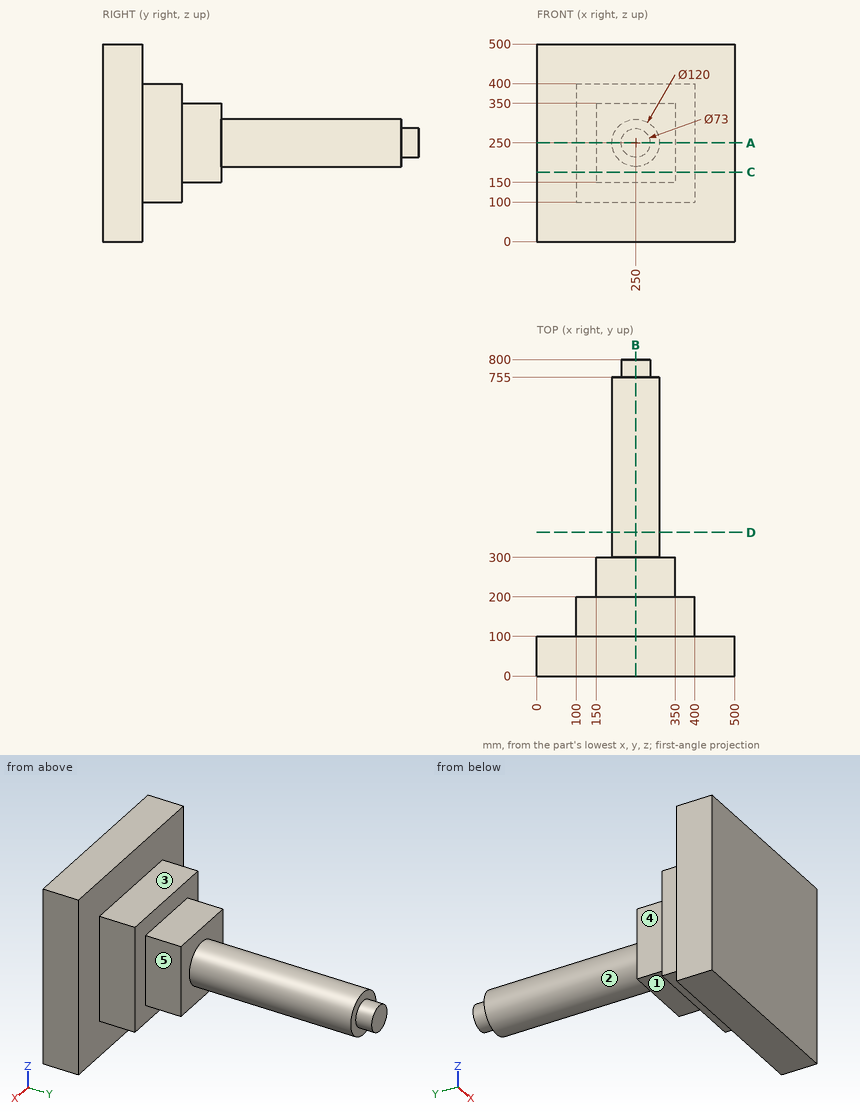
The drawing under review shows one solid part. Ordinate dimensions are in mm from its lowest x, y, z. A direction names the side the tool comes from. Give positions to 0.01 mm unless a question says otherwise; leave off trailing zeros. Write each loop counter-clockwise with the first axis right and the second up, starting at its lowest first coordinate (ties: lowest second). Pieces come first, ordered by that corner, then holes.
1. Tool access review of the marked faces 1, 2, 3, 4 and 5: name each direction out of +Z, -Z, +X, -X, +Y, -Y from which nothing blocks a thin tool from reaching the whole face with its end or side.
2. For P1, Ø10, axis at y = 220, z = 261, coming from the +X side; P2, Ø4, axis at x = 288.5, y = 178.5, coming from the -Z side; P3, Ø1.5, axis at x = 313.5, z = 431.5, coming from the +Y side, all flat-tipped, find the tip position at first contact; note any pin that passes through.
3. Add section D-D, the plane y = 363.5. Write out the cut boundary in (x, z).
4. Add section C-C, the plane z = 176. Write out the cut boundary in (x, y), plus the area to 3 significant figures.
5. Wall thickness on L1, parallel to Y at x = 45.5, z = 466.5; L2, parallel to Y at x = 306, z = 387.5; L3, parallel to X at y = 242.5, z = 281.5: over which ranges is each line inside the solid? List them lowest first.
6. Add section B-B, the plane x = 250. Write out the cut boundary in (y, z).
7. Add section A-A, the plane z = 250. Write out the cut boundary in (x, y).
Worked answers:
1. face 1: -Z, +X, -X, +Y
1. face 2: +Y
1. face 3: +Z, +X, -X, +Y
1. face 4: +Z, -Z, -X, +Y
1. face 5: +Z, -Z, +X, +Y
2. P1: stops at x = 350
2. P2: stops at z = 100
2. P3: stops at y = 100
3. outline: circle Ø120 at (250, 250)
4. outline: (0, 0) - (500, 0) - (500, 100) - (400, 100) - (400, 200) - (350, 200) - (350, 300) - (150, 300) - (150, 200) - (100, 200) - (100, 100) - (0, 100) - close
4. area: 100,000 mm2
5. L1: y = 0 to 100
5. L2: y = 0 to 200
5. L3: x = 150 to 350
6. outline: (0, 0) - (100, 0) - (100, 100) - (200, 100) - (200, 150) - (300, 150) - (300, 190) - (755, 190) - (755, 213.5) - (800, 213.5) - (800, 286.5) - (755, 286.5) - (755, 310) - (300, 310) - (300, 350) - (200, 350) - (200, 400) - (100, 400) - (100, 500) - (0, 500) - close
7. outline: (0, 0) - (500, 0) - (500, 100) - (400, 100) - (400, 200) - (350, 200) - (350, 300) - (310, 300) - (310, 755) - (286.5, 755) - (286.5, 800) - (213.5, 800) - (213.5, 755) - (190, 755) - (190, 300) - (150, 300) - (150, 200) - (100, 200) - (100, 100) - (0, 100) - close
